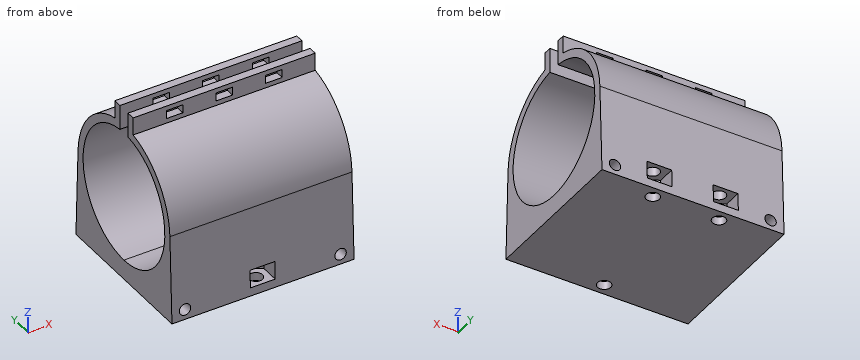
```python
from build123d import *

# Parameters (mm, degrees)
SKETCH1_R               = 28.575
SKETCH1_R_2             = 25.4
BOSS_EXTRUDE1_DEPTH     = 69.85
BOSS_EXTRUDE2_DEPTH     = 69.85
SKETCH4_R               = 2.5527
CUT_EXTRUDE1_DEPTH      = 16.256
CUT_EXTRUDE2_DEPTH      = 6.858
SKETCH9_W               = 9.949702626
SKETCH9_H               = 5.08
CUT_EXTRUDE3_DEPTH      = 83.825520976
BOSS_EXTRUDE3_DEPTH     = 69.85
SKETCH11_W              = 6.35
SKETCH11_H              = 3.175
CUT_EXTRUDE4_DEPTH      = 86.763649601
CUT_EXTRUDE5_DEPTH      = 84.332323558
CUT_EXTRUDE5_DEPTH_BACK = 84.332323558
SKETCH13_R              = 2.1844


with BuildPart() as part:
    # Sketch1 → Boss-Extrude1 (new body)
    with BuildSketch(Plane(origin=(0, 0, 0), x_dir=(0, 0, -1), z_dir=(1, 0, 0))):
        Circle(SKETCH1_R)
        Circle(SKETCH1_R_2, mode=Mode.SUBTRACT)
    extrude(amount=BOSS_EXTRUDE1_DEPTH)

    # Sketch2 → Boss-Extrude2 (add, through all)
    with BuildSketch(Plane(origin=(69.85, 0, 0), x_dir=(0, 0, -1), z_dir=(1, 0, 0))):
        with BuildLine():
            Line((33.02, -29.845), (33.02, 29.845))
            Line((33.02, 29.845), (-1.080565529, 28.554561862))
            ThreePointArc((-1.080565529, 28.554561862), (28.575, 0), (-1.080565529, -28.554561862))
            Line((-1.080565529, -28.554561862), (33.02, -29.845))
        make_face()
    extrude(amount=-BOSS_EXTRUDE2_DEPTH)

    # Sketch4 → Cut-Extrude1 (cut)
    with BuildSketch(Plane(origin=(0, 0, -33.02), x_dir=(-1, 0, 0), z_dir=(0, 0, -1))):
        with Locations((-47.625, 25.4)):
            Circle(SKETCH4_R)
        with Locations((-22.225, 25.4)):
            Circle(SKETCH4_R)
        with Locations((-34.925, -25.4)):
            Circle(SKETCH4_R)
    extrude(amount=-CUT_EXTRUDE1_DEPTH, mode=Mode.SUBTRACT)

    # Sketch7 → Cut-Extrude2 (cut)
    with BuildSketch(Plane(origin=(0, 0, -29.845), x_dir=(-1, 0, 0), z_dir=(0, 0, -1))):
        Polygon((-47.625, 19.900738686), (-42.8625, 22.650369343), (-42.8625, 29.845), (-45.79896584, 29.845), (-49.45103416, 29.845), (-52.3875, 29.845), (-52.3875, 22.650369343), align=None)
        Polygon((-24.05103416, 29.845), (-26.9875, 29.845), (-26.9875, 22.650369343), (-22.225, 19.900738686), (-17.4625, 22.650369343), (-17.4625, 29.845), (-20.39896584, 29.845), align=None)
        Polygon((-39.6875, -22.650369343), (-39.6875, -29.845), (-36.75103416, -29.845), (-33.09896584, -29.845), (-30.1625, -29.845), (-30.1625, -22.650369343), (-34.925, -19.900738686), align=None)
    extrude(amount=-CUT_EXTRUDE2_DEPTH, mode=Mode.SUBTRACT)

    # Sketch9 → Cut-Extrude3 (cut, through all)
    with BuildSketch(Plane(origin=(69.85, 0, 0), x_dir=(0, 0, -1), z_dir=(1, 0, 0))):
        with Locations((-25.4, 0)):
            Rectangle(SKETCH9_W, SKETCH9_H)
    extrude(amount=-CUT_EXTRUDE3_DEPTH, mode=Mode.SUBTRACT)

    # Sketch10 → Boss-Extrude3 (add, through all)
    with BuildSketch(Plane(origin=(69.85, 0, 0), x_dir=(0, 0, -1), z_dir=(1, 0, 0))):
        with BuildLine():
            Line((-34.811887235, 2.54), (-28.461887235, 2.54))
            ThreePointArc((-28.461887235, 2.54), (-28.274378752, 4.134021188), (-27.99766776, 5.715))
            Line((-27.99766776, 5.715), (-34.811887235, 5.715))
            Line((-34.811887235, 5.715), (-34.811887235, 2.54))
        make_face()
        with BuildLine():
            ThreePointArc((-27.99766776, -5.715), (-28.274378752, -4.134021188), (-28.461887235, -2.54))
            Line((-28.461887235, -2.54), (-34.811887235, -2.54))
            Line((-34.811887235, -2.54), (-34.811887235, -5.715))
            Line((-34.811887235, -5.715), (-27.99766776, -5.715))
        make_face()
    extrude(amount=-BOSS_EXTRUDE3_DEPTH)

    # Sketch11 → Cut-Extrude4 (cut, through all)
    with BuildSketch(Plane(origin=(0, 5.715, 0), x_dir=(1, 0, 0), z_dir=(0, 1, 0))):
        with Locations((53.975, -31.404777498)):
            Rectangle(SKETCH11_W, SKETCH11_H)
        with Locations((34.925, -31.404777498)):
            Rectangle(SKETCH11_W, SKETCH11_H)
        with Locations((15.875, -31.404777498)):
            Rectangle(SKETCH11_W, SKETCH11_H)
    extrude(amount=-CUT_EXTRUDE4_DEPTH, mode=Mode.SUBTRACT)

    # Sketch13 → Cut-Extrude5 (cut, two sides: drawn at the far end of the back side and taken through both)
    with BuildSketch(Plane(origin=(0, 0, 0.540476051), x_dir=(1, 0, 0), z_dir=(0, -1, 0)).offset(-CUT_EXTRUDE5_DEPTH_BACK)):
        with Locations(Location((64.77, -29.750476051, 0), (0, 0, 270))):
            Circle(SKETCH13_R)
        with Locations(Location((5.08, -29.750476051, 0), (0, 0, 270))):
            Circle(SKETCH13_R)
    extrude(amount=CUT_EXTRUDE5_DEPTH + CUT_EXTRUDE5_DEPTH_BACK, mode=Mode.SUBTRACT)


solid = part.part
```
Part model, mm, in its own coordinate system. Give positions to 0.01 mm unless a question says otherwise; leave off trailing zeros. Write each loop counter-clockwise with the first axis right and the second up, starting at its lowest first coordinate (ties: lowest second). Pieces come first, ordered by that corner, then holes. Notation, with made-up numbers: (-31.75, -35) -> (23.25, -35) arc R25 ccw to (23.25, -22) -> close; hole circle Ø7 at (58, 49.5). An arc over 180 degrees is marked (long way). Put each result on its own line as item: value. Start each with the question number.
Item 1: Pin check, flat tips, straight feed: pin 1 Ø1.5 at (x, z) = (8.5, 25) entering from +Y; pin 2 Ø5 at (x, y) = (50, 11.5) entering from +Z; pin 3 Ø5.5 at (x, z) = (64.77, -29.21) entering from +Y. Stop position of each tip, or through.
Item 2: Wall check: L1, parallel to X at y = 11.5, z = -29.21; L2, parallel to X at y = -16, z = -29; L3, parallel to X at y = -23, z = -26. Give the ranges that are in metal, low to high. Write a range as [from, to].
Item 3: Cut at D-D (z = 20). List the corners of the cut face in (x, y).
Item 4: Cut at A-A (y = -4). List the corners of the cut face in (x, z).
Item 5: Cut at B-B (x = 55). List the corners of the cut face in (y, z) (3 decimals).
Item 6: Cut at C-C (y = 15). List the corners of the cut face in (x, z).
Answer list:
1. pin 1: stops at y = 15.12
1. pin 2: stops at z = 27.12
1. pin 3: stops at y = 29.8
2. L1: x = [0, 2.9], [7.26, 62.59], [66.95, 69.85]
2. L2: x = [0, 2.91], [7.25, 62.6], [66.94, 69.85]
2. L3: x = [0, 30.16], [39.69, 69.85]
3. outline: (0, -20.41) -> (69.85, -20.41) -> (69.85, -15.66) -> (0, -15.66) -> close; (0, 15.66) -> (69.85, 15.66) -> (69.85, 20.41) -> (0, 20.41) -> close
4. outline: (0, -33.02) -> (69.85, -33.02) -> (69.85, -25.08) -> (0, -25.08) -> close; (0, 25.08) -> (69.85, 25.08) -> (69.85, 34.81) -> (0, 34.81) -> close; hole circle Ø4.37 at (5.08, -29.21); hole (12.7, 29.82) -> (19.05, 29.82) -> (19.05, 32.99) -> (12.7, 32.99) -> close; hole (31.75, 29.82) -> (38.1, 29.82) -> (38.1, 32.99) -> (31.75, 32.99) -> close; hole (50.8, 29.82) -> (57.15, 29.82) -> (57.15, 32.99) -> (50.8, 32.99) -> close; hole circle Ø4.37 at (64.77, -29.21)
5. outline: (-29.845, -33.02) -> (29.845, -33.02) -> (28.555, 1.081) arc R28.575 ccw to (5.715, 27.998) -> (5.715, 29.817) -> (2.54, 29.817) -> (2.54, 25.273) arc R25.4 cw (long way) to (-2.54, 25.273) -> (-2.54, 29.817) -> (-5.715, 29.817) -> (-5.715, 27.998) arc R28.575 ccw to (-28.555, 1.081) -> close; (-5.715, 32.992) -> (-2.54, 32.992) -> (-2.54, 34.812) -> (-5.715, 34.812) -> close; (2.54, 32.992) -> (5.715, 32.992) -> (5.715, 34.812) -> (2.54, 34.812) -> close
6. outline: (0, -33.02) -> (69.85, -33.02) -> (69.85, -20.5) -> (0, -20.5) -> close; (0, 20.5) -> (69.85, 20.5) -> (69.85, 24.32) -> (0, 24.32) -> close; hole circle Ø4.37 at (5.08, -29.21); hole circle Ø4.37 at (64.77, -29.21)
